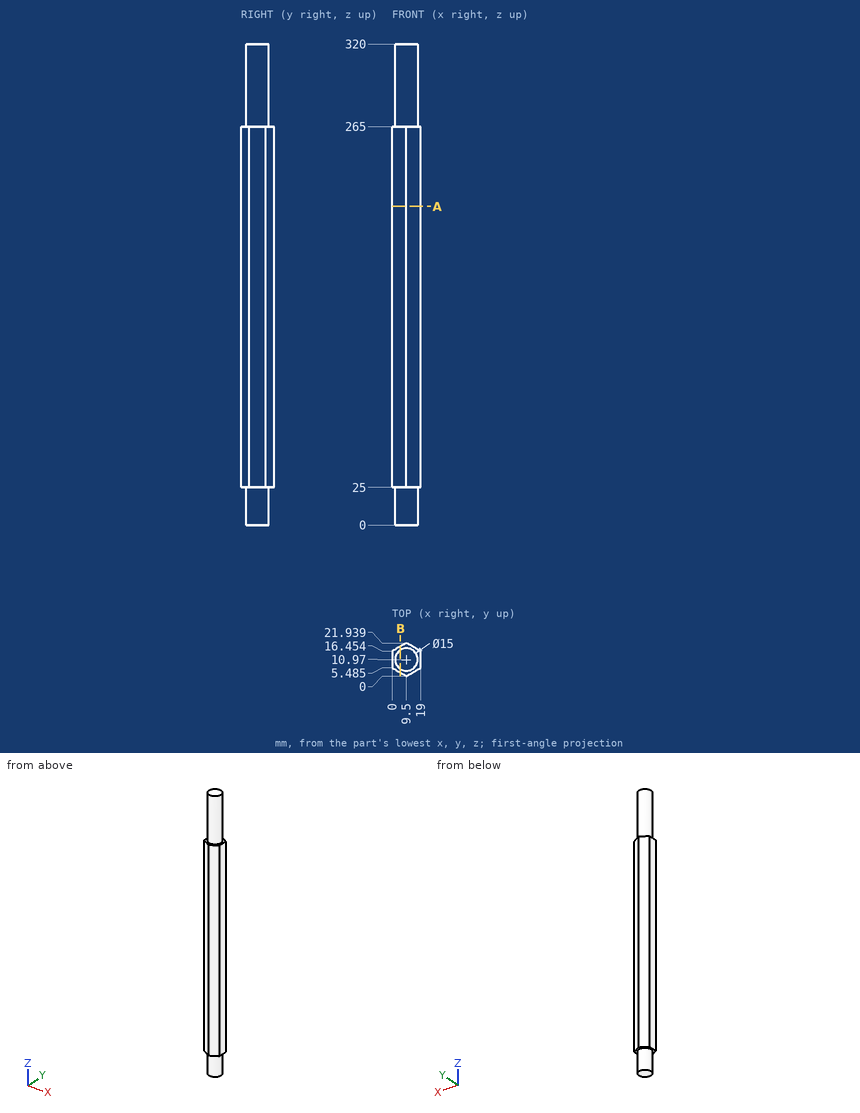
The figure shows three views and two pictorial views of one solid part (mm, origin at its lowest corner). Answer the questions. Round coordinates to 2 decimals unless told otherwise and drop trailing zeros. Order: outer loops, then holes, each group sorted by start corner. A loop starts at its lowest first (then second) coordinate and runs counter-clockwise, first axis right, second up. Notation, with made-up numbers: M 19,25.5 L 43,25.5 A7 ccw 43,31.5 Z; hole C 33.5,-3 d6. An arc over 180 degrees is marked long. Answer in a Markdown table with one row per item. Add a question column.
1) The part is cut by section B-B on x = 5.5. Determine the outline of the cut face in (y, z) (1 decimal), plus the area to 3 significant figures.
2) The part is cut by section A-A on z = 212. Determine the outline of the cut face in (x, y) (1 decimal), plus the area to 3 significant figures.
3) Flat-ended cylindrical pins translate along their axes: pin 1 Ø6 at (y, z) = (16.5, 268.5) entering from +X; pin 2 Ø5 at (x, z) = (10, 113) entering from +Y; pin 3 Ø3 at (x, z) = (7, 271.5) entering from +Y. Find the tip coordinate at first contact, or state that the pin passes through.
4) Consider line 1 along Z through (x, y) = (2.75, 7.5); line 2 along X through (y, z) = (11, 300); line 3 along Y through (x, z) = (3.5, 261) (1 decimal). Determine where each line is inside the solid, lowest interval first. Write a range as from..to.
Findings below:
| question | item | result |
|---|---|---|
| 1 | outline | M 2.3,25 L 4.6,25 L 4.6,0 L 17.3,0 L 17.3,25 L 19.6,25 L 19.6,265 L 17.3,265 L 17.3,320 L 4.6,320 L 4.6,265 L 2.3,265 Z |
| 1 | area | 5,170 mm² |
| 2 | outline | M 0,5.5 L 9.5,0 L 19,5.5 L 19,16.5 L 9.5,21.9 L 0,16.5 Z |
| 2 | area | 313 mm² |
| 3 | pin 1 | stops at x = 16.56 |
| 3 | pin 2 | stops at y = 21.94 |
| 3 | pin 3 | stops at y = 18.4 |
| 4 | line 1 | z = 25..265 |
| 4 | line 2 | x = 2..17 |
| 4 | line 3 | y = 3.5..18.5 |
